from build123d import *

# Parameters (mm, degrees)
F0_W     = 114.3
F0_H     = 139.7
F1_DEPTH = 46.99
F3_D     = 22.5044
F4_R     = 17.4625
F5_DEPTH = 133.35
F7_DEPTH = 139.701
F8_R     = 1.5875


with BuildPart() as f1:
    # F0 (on Top) → F1 (new body)
    with BuildSketch(Plane.XY):
        Rectangle(F0_W, F0_H)
    extrude(amount=F1_DEPTH)

    # F3 (through all)
    with Locations(Plane.XZ.offset(69.85)):
        with Locations((-33.655, 23.495), (33.655, 23.495)):
            Hole(F3_D / 2)

    # F4 (on face) → F5 (cut, through all)
    with BuildSketch(Plane.XZ.offset(69.85)):
        with Locations((0, 23.495)):
            Circle(F4_R)
    extrude(amount=-F5_DEPTH, mode=Mode.SUBTRACT)

    # F6 (on face) → F7 (cut, through all)
    with BuildSketch(Plane.XZ.offset(69.85)):
        with BuildLine():
            Line((-50.9913984587, 37.4018297423), (-57.15, 40.9575))
            Line((-57.15, 40.9575), (-57.15, 6.0325))
            Line((-57.15, 6.0325), (-50.9913984587, 9.5881702577))
            ThreePointArc((-50.9913984587, 9.5881702577), (-55.88, 23.495), (-50.9913984587, 37.4018297423))
        make_face()
        Polygon((-22.5425, 46.99), (-44.7675, 46.99), (-42.017869343, 42.2275), (-25.292130657, 42.2275), align=None)
        Polygon((-42.017869343, 4.7625), (-44.7675, 0), (-22.5425, 0), (-25.292130657, 4.7625), align=None)
        with BuildLine():
            Line((-12.800001213, 5.3260541322), (-15.875, 0))
            Line((-15.875, 0), (15.875, 0))
            Line((15.875, 0), (12.800001213, 5.3260541322))
            ThreePointArc((12.800001213, 5.3260541322), (0, 1.27), (-12.800001213, 5.3260541322))
        make_face()
        with BuildLine():
            Line((15.875, 46.99), (-15.875, 46.99))
            Line((-15.875, 46.99), (-12.800001213, 41.6639458678))
            ThreePointArc((-12.800001213, 41.6639458678), (0, 45.72), (12.800001213, 41.6639458678))
            Line((12.800001213, 41.6639458678), (15.875, 46.99))
        make_face()
        Polygon((44.7675, 46.99), (22.5425, 46.99), (25.292130657, 42.2275), (42.017869343, 42.2275), align=None)
        Polygon((25.292130657, 4.7625), (22.5425, 0), (44.7675, 0), (42.017869343, 4.7625), align=None)
        with BuildLine():
            Line((57.15, 6.0325), (57.15, 40.9575))
            Line((57.15, 40.9575), (50.9913984587, 37.4018297423))
            ThreePointArc((50.9913984587, 37.4018297423), (55.88, 23.495), (50.9913984587, 9.5881702577))
            Line((50.9913984587, 9.5881702577), (57.15, 6.0325))
        make_face()
    extrude(amount=-F7_DEPTH, mode=Mode.SUBTRACT)

    # F8
    f8_edges = [f1.edges().sort_by_distance(p)[0] for p in [
        (-57.15, 0, 0),
        (-44.7675, 0, 0),
        (-42.017869, 0, 4.7625),
        (-25.292131, 0, 4.7625),
        (-22.5425, 0, 0),
        (-15.875, 0, 0),
        (-12.800001, 0, 5.326054),
        (12.800001, 0, 5.326054),
        (15.875, 0, 0),
        (22.5425, 0, 0),
        (25.292131, 0, 4.7625),
        (42.017869, 0, 4.7625),
        (44.7675, 0, 0),
        (57.15, 0, 0),
        (57.15, 0, 6.0325),
        (50.991398, 0, 37.40183),
        (50.991398, 0, 9.58817),
        (57.15, 0, 46.99),
        (44.7675, 0, 46.99),
        (42.017869, 0, 42.2275),
        (25.292131, 0, 42.2275),
        (22.5425, 0, 46.99),
        (15.875, 0, 46.99),
        (12.800001, 0, 41.663946),
        (-12.800001, 0, 41.663946),
        (-15.875, 0, 46.99),
        (-22.5425, 0, 46.99),
        (-25.292131, 0, 42.2275),
        (-42.017869, 0, 42.2275),
        (-44.7675, 0, 46.99),
        (-57.15, 0, 46.99),
        (-57.15, 0, 40.9575),
        (-50.991398, 0, 37.40183),
        (-50.991398, 0, 9.58817),
        (-57.15, 0, 6.0325),
    ]]
    fillet(f8_edges, radius=F8_R)


solid = f1.part
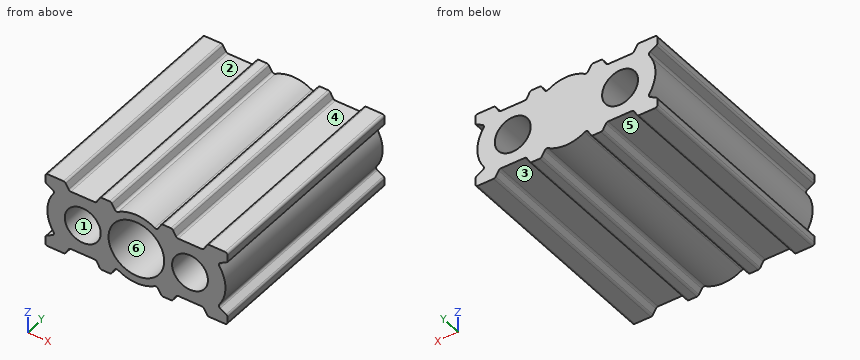
Geometry: final body of the model. Coordinates: model frame, mm. Face numbers are marked on the shaded views. A direction names the side the tool comes from. Coordinates: 2 decimals unless noted, no trailing zeros. Loops run counter-clockwise (first coordinate to the right, second up) from the corner with the lowest first, then second, coordinate; pieces in that order, holes last. Notation, with made-up numbers: (-24, 76.25) - (28, 76.25) arc R33 ccw to (28, 115.25) - close; hole circle Ø1 at (10, -27.5). An arc over 180 degrees is marked (long way). Put each result on its own line as item: value. Start each with the question number.
Q1. Cut plane B-B, the plane x = 0. Return loops of the section in (y, z).
Q2. Cut plane C-C, the plane z = 15. Return loops of the section in (x, y).
Q3. Set-up query: the marked faces 4, 5 and 6. Return all of +Z, -Z, +X, -X, +Y, -Y with unobstructed straight access to the full face (end or side cutting, diameter ignored); none if empty.
Q4. Pin query (flat end, axial travel): pin 1 Ø8 at (x, z) = (0.5, 7) entering from -Y; pin 2 Ø12 at (x, y) = (-37.5, 26.5) entering from +Z; pin 3 Ø12 at (x, y) = (-10, 37) entering from -Z; pin 4 Ø10 at (x, y) = (-37, 31.5) entering from +Z. Return the tip coordinate at first contact, or that it passes through.
Q5. Line query: line 1 (Z direction, x = 0, y = 3); line 2 (Z direction, x = -34, y = 13.5); line 3 (X direction, y = 54, z = 30). Output: solid intervals per line, ascending.
Q6. Pull-direction query (Z, two-part tool) for the marked faces 1, 2 and 3; classes: released by +Z, released by -Z, zero draft, split by the parting line, or undercut.
Q7. Cut plane A-A, the plane z = 22. Return loops of the section in (x, y).
Q8. Cut plane D-D, the plane y = 36.5. Give the number of separate pieces and of enclosed holes in the cut face, and give its area (3 significant figures).
Filled sheet:
1. outline: (-69.85, 1.27) - (69.85, 1.27) - (69.85, 45.72) - (-69.85, 45.72) - (-69.85, 40.96) - (63.5, 40.96) - (63.5, 6.03) - (-69.85, 6.03) - close
2. outline: (-54.19, -69.85) - (-41.03, -69.85) - (-41.03, 69.85) - (-54.19, 69.85) - close; (-26.28, -69.85) - (-15.26, -69.85) - (-15.26, 63.5) - (15.26, 63.5) - (15.26, -69.85) - (26.28, -69.85) - (26.28, 69.85) - (-26.28, 69.85) - close; (41.03, -69.85) - (54.19, -69.85) - (54.19, 69.85) - (41.03, 69.85) - close
3. face 4: +Z, +Y, -Y
3. face 5: -Z, +Y, -Y
3. face 6: -Y
4. pin 1: y = -69.85
4. pin 2: z = 44.79
4. pin 3: z = 0.21
4. pin 4: z = 42.51
5. line 1: 1.27 to 6.03, 40.96 to 45.72
5. line 2: 4.76 to 12.25, 34.74 to 42.23
5. line 3: -54.91 to -42.84, -24.47 to -16.21, 16.21 to 24.47, 42.84 to 54.91
6. face 1: undercut
6. face 2: released by +Z
6. face 3: released by -Z
7. outline: (-55.83, -69.85) - (-44.81, -69.85) - (-44.81, 69.85) - (-55.83, 69.85) - close; (-22.5, -69.85) - (-17.4, -69.85) - (-17.4, 63.5) - (17.4, 63.5) - (17.4, -69.85) - (22.5, -69.85) - (22.5, 69.85) - (-22.5, 69.85) - close; (44.81, -69.85) - (55.83, -69.85) - (55.83, 69.85) - (44.81, 69.85) - close
8. separate pieces: 1
8. enclosed holes: 3
8. area: 2,880 mm²
